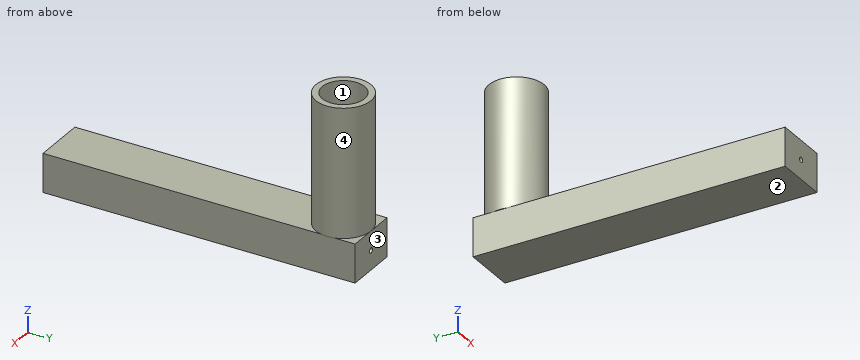
```python
from build123d import *

# Parameters (mm, degrees)
SKETCH_1_R          = 10.75
EXTRUDE_1_DEPTH     = 50
SKETCH_2_W          = 20.887285672
SKETCH_2_H          = 21.5
EXTRUDE_2_DEPTH     = 15
SKETCH_3_W          = 20.887285672
SKETCH_3_H          = 15
EXTRUDE_3_DEPTH     = 100
SKETCH_4_R          = 1
CUT_EXTRUDE_1_DEPTH = 130
SKETCH_5_R          = 8.25
CUT_EXTRUDE_4_DEPTH = 50


with BuildPart() as part:
    # Sketch 1 → Extrude 1 (new body)
    with BuildSketch(Plane.XY):
        Circle(SKETCH_1_R)
    extrude(amount=EXTRUDE_1_DEPTH)

    # Sketch 2 → Extrude 2 (add)
    with BuildSketch(Plane.XY):
        Rectangle(SKETCH_2_W, SKETCH_2_H)
    extrude(amount=-EXTRUDE_2_DEPTH)

    # Sketch 3 → Extrude 3 (add)
    with BuildSketch(Plane.XZ.offset(10.75)):
        with Locations((0, -7.5)):
            Rectangle(SKETCH_3_W, SKETCH_3_H)
    extrude(amount=EXTRUDE_3_DEPTH)

    # Sketch 4 → Cut-Extrude 1 (cut)
    with BuildSketch(Plane(origin=(0, 10.75, 0), x_dir=(1, 0, 0), z_dir=(0, 1, 0))):
        with Locations(Location((0, 7.5, 0), (0, 0, 180))):
            Circle(SKETCH_4_R)
    extrude(amount=-CUT_EXTRUDE_1_DEPTH, mode=Mode.SUBTRACT)

    # Sketch 5 → Cut-Extrude 4 (cut)
    with BuildSketch(Plane.XY.offset(50)):
        Circle(SKETCH_5_R)
    extrude(amount=-CUT_EXTRUDE_4_DEPTH, mode=Mode.SUBTRACT)


solid = part.part
```
Check sheet for the modelled part. Datum: model origin and axes. Units: mm. Face numbers are marked on the shaded views. Coordinates: 2 decimals unless noted, no trailing zeros. Order: outer loops, then holes, each group sorted by start corner. A loop starts at its lowest first (then second) coordinate and runs counter-clockwise, first axis right, second up. Notation, with made-up numbers: (32, -33.75) -> (67, -33.75) arc R23 ccw to (67, 2.25) -> close; hole circle Ø7 at (-4.75, -2). An arc over 180 degrees is marked (long way). Write each question's results on one line, items separated by ' | '. Start each with the question number.
1) Material ranges on line 1 along Y through (x, z) = (0, 37.5); line 2 along Z through (x, y) = (0, -17); line 3 along Z through (x, y) = (-4.5, -77.5), recorded low to high.
2) Section check B-B (x = 4.25). Enter the section's corners in (y, z), and give its area (3 significant figures).
3) Section check D-D (y = -98). Enter the section's corners in (x, z).
4) Draft check along Y on the marked faces 1, 2, 3 and 4. Enter one of: pulls with the +Y half, pulls with the -Y half, needs draft (parallel to the pull), parting line crosses it, or undercut.
5) Section check A-A (y = 0). Enter the section's corners in (x, z), and give its area (3 significant figures).
6) Section check C-C (z = 38). Enter the section's corners in (x, y).
7) Depth check by flat-ended pin: pin 1 (6 mm diameter, centred on x = -7, z = 33.5, fed in from -Y); pin 2 (9 mm diameter, centred on x = -2.5, y = 6, fed in from +Z); pin 3 (12 mm diameter, centred on y = -64.5, z = -5, fed in from -X); pin 4 (6.5 mm diameter, centred on x = 3.5, y = -66, fed in from +Z). Enter the tip coordinate at first touch or a pass-through.
Checked values:
1) line 1: -10.75 to -8.25, 8.25 to 10.75 | line 2: -15 to -8.5, -6.5 to 0 | line 3: -15 to 0
2) outline: (-110.75, -15) -> (10.75, -15) -> (10.75, 0) -> (9.87, 0) -> (9.87, 50) -> (7.07, 50) -> (7.07, 0) -> (-7.07, 0) -> (-7.07, 50) -> (-9.87, 50) -> (-9.87, 0) -> (-110.75, 0) -> close | area: 2,100 mm²
3) outline: (-10.44, -15) -> (10.44, -15) -> (10.44, 0) -> (-10.44, 0) -> close; hole circle Ø2 at (0, -7.5)
4) face 1: undercut | face 2: needs draft | face 3: pulls with the +Y half | face 4: parting line crosses it
5) outline: (-10.75, 0) -> (-10.44, 0) -> (-10.44, -15) -> (10.44, -15) -> (10.44, 0) -> (10.75, 0) -> (10.75, 50) -> (8.25, 50) -> (8.25, 0) -> (-8.25, 0) -> (-8.25, 50) -> (-10.75, 50) -> close; hole circle Ø2 at (0, -7.5) | area: 560 mm²
6) outline: circle Ø21.5 at (0, 0); hole circle Ø16.5 at (0, 0)
7) pin 1: y = -9.98 | pin 2: z = 50 | pin 3: x = -10.44 | pin 4: z = 0
